Could you check a few things on this model? Use its own coordinates, in mm. A direction names the side the tool comes from. Round coordinates to 2 decimals unless told otherwise and drop trailing zeros. Loops run counter-clockwise (first coordinate to the right, second up) from the corner with the lowest first, then second, coordinate; pieces in that order, holes last. Notation, with made-up numbers: (56.25, -12) -> (111.25, -12) arc R10 cw to (111.25, 5) -> close; hole circle Ø8 at (16, -29). An arc over 180 degrees is marked (long way). One line per item, written item: value.
```python
from build123d import *

# Parameters (mm, degrees)
F0_W     = 1.5
F0_H     = 1
F0_H_2   = 7
F1_DEPTH = 2
F2_DEPTH = 0.25
F3_R     = 0.74999
F4_R     = 0.3


# Not quite as in the source:
# - a fillet or chamfer is up to 0.001 mm smaller than in the source, because OpenCascade refuses the exact size
# - a feature names something its author has since deleted; it is built from what else it names


with BuildPart() as f1:
    # F0 (on Top) → F1 (new body)
    with BuildSketch(Plane.XY):
        with Locations((-0.75, 9.1787409857)):
            Rectangle(F0_W, F0_H)
        with Locations((-0.75, 5.1787409857)):
            Rectangle(F0_W, F0_H_2)
        with Locations((-0.75, 1.1787409857)):
            Rectangle(F0_W, F0_H)
    extrude(amount=F1_DEPTH)

    # F0 (on Top) → F2 (join)
    with BuildSketch(Plane.XY):
        with Locations((-0.75, 1.1787409857)):
            Rectangle(F0_W, F0_H)
        Polygon((-1.5, 0.6787409857), (-1.5, 1.6787409857), (-1.9, 1.6787409857), (-1.9, 0.1787409857), (0.4, 0.1787409857), (0.4, 1.6787409857), (0, 1.6787409857), (0, 0.6787409857), align=None)
        Polygon((-1.5, 8.6787409857), (-1.5, 9.6787409857), (0, 9.6787409857), (0, 8.6787409857), (0.4, 8.6787409857), (0.4, 10.1787409857), (-1.9, 10.1787409857), (-1.9, 8.6787409857), align=None)
        with Locations((-0.75, 9.1787409857)):
            Rectangle(F0_W, F0_H)
    extrude(amount=-F2_DEPTH)

    # F3 (radius 0.75 in the source; OpenCascade refuses exactly that, so slightly less here)
    f3_edges = [f1.edges().sort_by_distance(p)[0] for p in [
        (0, 9.678741, 1),
        (-1.5, 9.678741, 1),
        (0, 0.678741, 1),
        (-1.5, 0.678741, 1),
    ]]
    fillet(f3_edges, radius=F3_R)

    # F4
    f4_edges = [f1.edges().sort_by_distance(p)[0] for p in [
        (0.4, 10.178741, -0.125),
        (-1.9, 10.178741, -0.125),
        (0.4, 0.178741, -0.125),
        (-1.9, 0.178741, -0.125),
    ]]
    fillet(f4_edges, radius=F4_R)


solid = f1.part
```
Item 1: I need wall thicknesses on line 1 (Y direction, x = -1.6, z = -0.2); line 2 (Z direction, x = -1.35, y = 6.25); line 3 (X direction, y = 7.75, z = 0.55). Which ranges of each line are inside material? Lowest first, please. Write a range as from..to.
Output:
line 1: y = 0.18..1.68, 8.68..10.18
line 2: z = 0..2
line 3: x = -1.5..0
Item 2: Will this pin go through, and if not, where does the flat tip stop? pin 1 Ø0.8 at (x, y) = (-1, 6) entering from -Z.
Output:
pin 1: stops at z = 0
Item 3: If we section it at B-B on x = -1.4: List the corners of the cut face in (y, z) for me.
Output:
outline: (0.18, -0.25) -> (1.68, -0.25) -> (1.68, 0) -> (8.68, 0) -> (8.68, -0.25) -> (10.18, -0.25) -> (10.18, 0) -> (9.3, 0) -> (9.3, 2) -> (1.05, 2) -> (1.05, 0) -> (0.18, 0) -> close
Item 4: If we section it at D-D on x = -0.35: List the corners of the cut face in (y, z) for me, plus the area to 3 significant figures.
Output:
outline: (0.18, -0.25) -> (1.68, -0.25) -> (1.68, 0) -> (8.68, 0) -> (8.68, -0.25) -> (10.18, -0.25) -> (10.18, 0) -> (9.56, 0) -> (9.56, 2) -> (0.79, 2) -> (0.79, 0) -> (0.18, 0) -> close
area: 18.3 mm²
Item 5: If we section it at C-C on y = 5.25: List the corners of the cut face in (x, z) for me.
Output:
outline: (-1.5, 0) -> (0, 0) -> (0, 2) -> (-1.5, 2) -> close
Item 6: If we mould it in two halves opening along Y, with no side actions, what happens to faces 1 (the face through (-1, 10, 0)), 2 (the face through (-1, 5, 0))? For each: released by +Y, released by -Y, zero draft, split by the parting line, or undercut.
Output:
face 1: zero draft
face 2: undercut
Item 7: For faces 3 (the face through (-1, 5, 2)), 4 (the face through (-0.8, 0.4, 0)), which set-ups out of +Z, -Z, +X, -X, +Y, -Y let a thin tool reach every point of the face, with its end or its side?
Output:
face 3: +Z, +X, -X, +Y, -Y
face 4: +Z, -X, -Y
